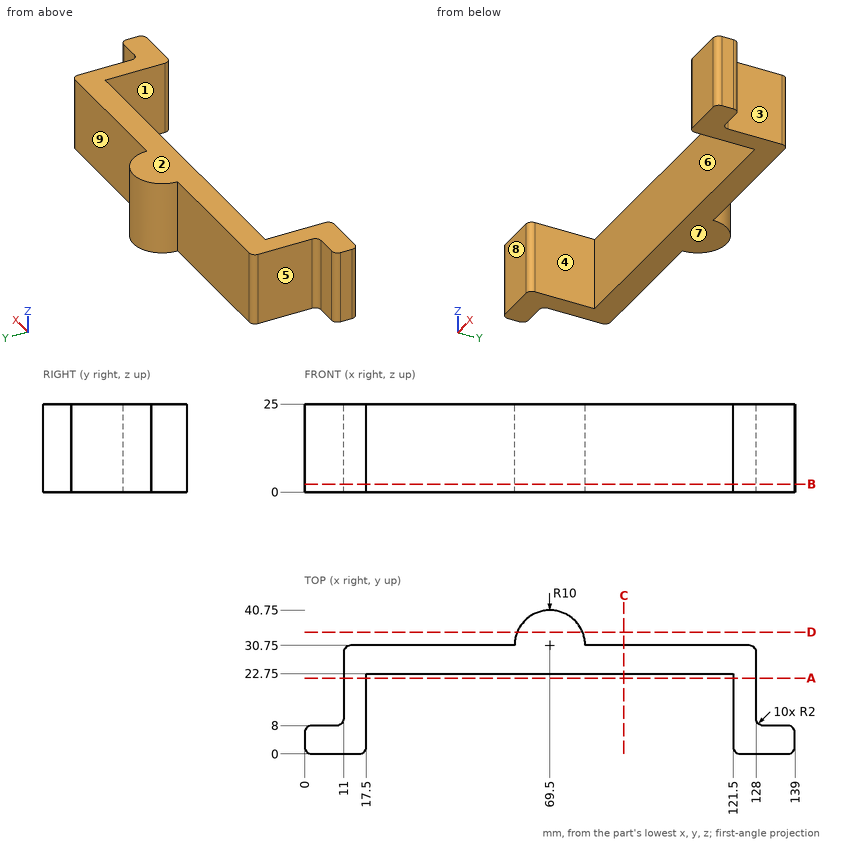
Here's the drawing with two shaded views (mm, measured from the low corner). I have some questions. A direction names the side the tool comes from. Coordinates: 2 decimals unless noted, no trailing zeros. Order: outer loops, then holes, each group sorted by start corner. A loop starts at its lowest first (then second) coordinate and runs counter-clockwise, first axis right, second up.
Q1. Which directions (+Z, -Z, +X, -X, +Y, -Y) give clear straight access to the entire face, cutting with the end or side of a thin tool? Please do the marked faces 5, 6, 7, 8 and 9.
Q2. Suppose I cut it at B-B on z = 2.25. Please give me the cut outline in (x, y).
Q3. Suppose I cut it at A-A on y = 21.5. Please give me the cut outline in (x, z).
Q4. Please list where these lines run through material, in increasing order: L1, parallel to X at y = 17, z = 7.25; L2, parallel to X at y = 4, z = 3.5; L3, parallel to Y at x = 105.5, z = 15.5.
Q5. Thinking about a two-plate mould opening in X: for the marked faces 1, 2, 3 and 4, which applies, released by +X, released by -X, zero draft, split by the parting line, or undercut?
Q6. Will these pins go through, and if not, where does the flat tip stop? pin 1 (1.5 mm diameter, centred on x = 85, z = 15, fed in from +Y); pin 2 (7.5 mm diameter, centred on x = 4.5, z = 16.5, fed in from +Y); pin 3 (4 mm diameter, centred on y = 28.5, z = 12.5, fed in from +X).
Q7. Suppose I cut it at C-C on x = 90.5. Please give me the cut outline in (y, z), and give its area (3 significant figures).
Q8. Suppose I cut it at D-D on y = 34.5. Please give me the cut outline in (x, z), and give its area (3 significant figures).
Answer:
1. face 5: +Z, -Z, -X, +Y
1. face 6: +Z, -Z, -Y
1. face 7: -Z, +X, -X, +Y, -Y
1. face 8: +Z, -Z, +X, -X, -Y
1. face 9: +Z, -Z, +X, +Y
2. outline: (0, 2) arc R2 ccw to (2, 0) - (15.5, 0) arc R2 ccw to (17.5, 2) - (17.5, 22.75) - (121.5, 22.75) - (121.5, 2) arc R2 ccw to (123.5, 0) - (137, 0) arc R2 ccw to (139, 2) - (139, 6) arc R2 ccw to (137, 8) - (130, 8) arc R2 cw to (128, 10) - (128, 28.75) arc R2 ccw to (126, 30.75) - (79.5, 30.75) arc R10 ccw to (59.5, 30.75) - (13, 30.75) arc R2 ccw to (11, 28.75) - (11, 10) arc R2 cw to (9, 8) - (2, 8) arc R2 ccw to (0, 6) - close
3. outline: (11, 0) - (17.5, 0) - (17.5, 25) - (11, 25) - close; (121.5, 0) - (128, 0) - (128, 25) - (121.5, 25) - close
4. L1: x = 11 to 17.5, 121.5 to 128
4. L2: x = 0 to 17.5, 121.5 to 139
4. L3: y = 22.75 to 30.75
5. face 1: undercut
5. face 2: zero draft
5. face 3: released by +X
5. face 4: undercut
6. pin 1: stops at y = 30.75
6. pin 2: stops at y = 8
6. pin 3: stops at x = 128
7. outline: (22.75, 0) - (30.75, 0) - (30.75, 25) - (22.75, 25) - close
7. area: 200 mm2
8. outline: (60.23, 0) - (78.77, 0) - (78.77, 25) - (60.23, 25) - close
8. area: 464 mm2
